Autodesk Inventor part; units mm, degrees
ref_plane "YZ Plane" through (0, 0, 0) normal (1, 0, 0) x (0, 1, 0)
ref_plane "XZ Plane" through (0, 0, 0) normal (0, 1, 0) x (-1, 0, 0)
ref_plane "XY Plane" through (0, 0, 0) normal (0, 0, 1) x (1, 0, 0)
sketch "Sketch1" plane through (0, 0, 0) normal (0, 0, 1) x (1, 0, 0)
  line L0 (-7.5, 10) -> (7.5, 10)
  line L1 (7.5, 10) -> (7.5, -10)
  line L2 (7.5, -10) -> (-7.5, -10)
  line L3 (-7.5, -10) -> (-7.5, 10)
  point P0 (0, 0)
  dimension "d0" = 15
  dimension "d1" = 20
  dimension "d2" = 7.5
  dimension "d3" = 10
extrude "Extrusion1" add sketch "Sketch1" along normal blind 1
fillet "Fillet1" radius 2 4 edges at (7.5, 10, 0.5) (-7.5, 10, 0.5) (7.5, -10, 0.5) (-7.5, -10, 0.5)
sketch "Sketch2" plane through (0, 0, 1) normal (0, 0, 1) x (1, 0, 0)
  line L0 (-5.5, -10) -> (5.5, -10)
  line L1 (5.5, 10) -> (-5.5, 10)
  line L2 (-7.5, 8) -> (-7.5, -8)
  line L3 (-4, 7.5) -> (4, 7.5)
  line L4 (4, 7.5) -> (4, 6.5)
  line L5 (4, 6.5) -> (-4, 6.5)
  line L6 (-4, 6.5) -> (-4, 7.5)
  line L7 (-4, 2.5) -> (4, 2.5)
  line L8 (4, 2.5) -> (4, 1.5)
  line L9 (4, 1.5) -> (-4, 1.5)
  line L10 (-4, 1.5) -> (-4, 2.5)
  circle A0 centre (0, -5) radius 2.625
  point P0 (0, 0)
  dimension "d7" = 8
  dimension "d8" = 1
  dimension "d9" = 3.5
  dimension "d10" = 2.5
  dimension "d11" = 1
  dimension "d12" = 4
  dimension "d13" = 3.5
  dimension "d14" = 8
  dimension "d15" = 5.25
  dimension "d16" = 5
  dimension "d17" = 7.5
extrude "Extrusion2" cut sketch "Sketch2" against normal through all
properties part number "belt_clip" material "Nylon 6/6"
Geometry check sheet. Reference: the model listing, model coordinates, mm. A direction names the side the tool comes from. Round coordinates to 2 decimals unless told otherwise and drop trailing zeros. Order: outer loops, then holes, each group sorted by start corner. A loop starts at its lowest first (then second) coordinate and runs counter-clockwise, first axis right, second up. Notation, with made-up numbers: M -18.75,5 L 27.25,5 A32 cw 27.25,34 Z; hole C 11.5,47 d8. An arc over 180 degrees is marked long. Write each question's results on one line, items separated by ' | '. Start each with the question number.
1. Go/stop test with a flat-tipped pin: P1, Ø4.5, axis at x = 0, y = -5, coming from the +Z side. Record where the tip stops, or that it passes through.
2. Cross-section at A-A on y = -5. Record the boundary of the cut face in (x, z) (3 decimals).
3. Draft check along X on faces 3 (the face through (4, 2, 0.5)), 4 (the face through (7.5, 0.1, 0.5)), 5 (the face through (-6.9, 9.43, 0.51)). Enter one of: pulls with the +X half, pulls with the -X half, needs draft (parallel to the pull), parting line crosses it, or undercut.
4. Material ranges on L1, parallel to Y at x = 0, z = 0.3 (3 decimals); L2, parallel to Y at x = 3.75, z = 0.9; L3, parallel to Y at x = 1.5, z = 0.9, recorded low to high. Write a range as from..to.
5. Set-up check for faces 1 (the face through (-6.93, -9.4, 0.51)), 2 (the face through (-4, 7, 0.5)): record each of +Z, -Z, +X, -X, +Y, -Y from which the full face is reachable in a straight line by a thin tool's end or side.
6. Cross-section at B-B on x = 0. Record the boundary of the cut face in (y, z) (3 decimals), plus the area to 4 significant figures.
7. Cross-section at C-C on z = 0.2. Record the boundary of the cut face in (x, y) (3 decimals).
Resolved:
1) P1: through
2) outline: M -7.5,0 L -2.625,0 L -2.625,1 L -7.5,1 Z; M 2.625,0 L 7.5,0 L 7.5,1 L 2.625,1 Z
3) face 3: undercut | face 4: pulls with the +X half | face 5: pulls with the -X half
4) L1: -10..-7.625, -2.375..1.5, 2.5..6.5, 7.5..10 | L2: -10..1.5, 2.5..6.5, 7.5..10 | L3: -10..-7.15, -2.85..1.5, 2.5..6.5, 7.5..10
5) face 1: +Z, -Z, -X, -Y | face 2: +Z, -Z
6) outline: M -10,0 L -7.625,0 L -7.625,1 L -10,1 Z; M -2.375,0 L 1.5,0 L 1.5,1 L -2.375,1 Z; M 2.5,0 L 6.5,0 L 6.5,1 L 2.5,1 Z; M 7.5,0 L 10,0 L 10,1 L 7.5,1 Z | area: 12.75 mm2
7) outline: M -7.5,-8 A2 ccw -5.5,-10 L 5.5,-10 A2 ccw 7.5,-8 L 7.5,8 A2 ccw 5.5,10 L -5.5,10 A2 ccw -7.5,8 Z; hole M -4,1.5 L 4,1.5 L 4,2.5 L -4,2.5 Z; hole M -4,6.5 L 4,6.5 L 4,7.5 L -4,7.5 Z; hole C 0,-5 d5.25
